from build123d import *

# Parameters (mm, degrees)
SKETCH001_W       = 214
SKETCH001_H       = 314
PAD_DEPTH         = 3
SKETCH_W          = 4
SKETCH_H          = 15
SKETCH_W_2        = 2
SKETCH_H_2        = 4
PAD001_DEPTH      = 0.3
SKETCH002_R       = 1.5
SKETCH002_R_2     = 0.75
POCKET_DEPTH      = 3.001
POCKET_DEPTH_BACK = -0.301


with BuildPart() as part:
    # Sketch001 → Pad (new body)
    with BuildSketch(Plane(origin=(110.543777, 322.172485, 403.912964), x_dir=(0, -1, 0), z_dir=(0, 0, 1))):
        with Locations((-107, 157)):
            Rectangle(SKETCH001_W, SKETCH001_H)
    extrude(amount=PAD_DEPTH)

    # Sketch → Pad001 (new body)
    with BuildSketch(Plane(origin=(110.543777, 322.172485, 406.912964), x_dir=(0, -1, 0), z_dir=(0, 0, 1))):
        with Locations((-208, 140)):
            Rectangle(SKETCH_W, SKETCH_H)
        with Locations((-208, 180)):
            Rectangle(SKETCH_W, SKETCH_H)
        with Locations((-208, 198)):
            Rectangle(SKETCH_W, SKETCH_H)
        with Locations((-210, 162.5)):
            Rectangle(SKETCH_W_2, SKETCH_H_2)
        with Locations((-207, 162.5)):
            Rectangle(SKETCH_W_2, SKETCH_H_2)
        with Locations((-208, 166.51)):
            Rectangle(SKETCH_W_2, SKETCH_H_2)
    extrude(amount=PAD001_DEPTH)

    # Sketch002 → Pocket (cut, two sides)
    with BuildSketch(Plane(origin=(110.543777, 322.172485, 406.912964), x_dir=(0, -1, 0), z_dir=(0, 0, 1))) as pocket_sk:
        with Locations((-208, 139.5)):
            Circle(SKETCH002_R)
        with Locations((-211, 157)):
            Circle(SKETCH002_R)
        with Locations((-210, 161.5)):
            Circle(SKETCH002_R_2)
        with Locations((-210, 163.5)):
            Circle(SKETCH002_R_2)
        with Locations((-207, 161.5)):
            Circle(SKETCH002_R_2)
        with Locations((-207, 163.5)):
            Circle(SKETCH002_R_2)
        with Locations((-208, 167.5)):
            Circle(SKETCH002_R_2)
        with Locations((-208, 165.5)):
            Circle(SKETCH002_R_2)
        with Locations((-208, 180.5)):
            Circle(SKETCH002_R)
        with Locations((-208, 197.5)):
            Circle(SKETCH002_R)
        with Locations((-211, 311)):
            Circle(SKETCH002_R)
        with Locations((-211, 3)):
            Circle(SKETCH002_R)
        with Locations((-3, 3)):
            Circle(SKETCH002_R)
        with Locations((-3, 311)):
            Circle(SKETCH002_R)
        with BuildLine():
            Line((-109.25, 159.250001), (-109.25, 153.25))
            Line((-109.25, 153.25), (-106.25, 153.25))
            Line((-106.25, 159.25), (-106.25, 153.25))
            ThreePointArc((-106.25, 159.25), (-107.75, 160.749999), (-109.25, 159.250001))
        make_face()
    extrude(amount=-POCKET_DEPTH, mode=Mode.SUBTRACT)
    extrude(pocket_sk.sketch, amount=-POCKET_DEPTH_BACK, mode=Mode.SUBTRACT)


solid = part.part
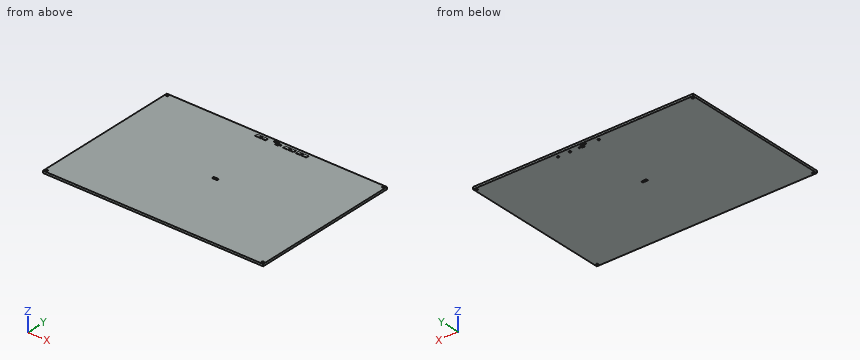
For this review, take the finished solid that the model builds, in its own axes (mm). Give positions to 0.01 mm unless a question says otherwise; leave off trailing zeros. Order: outer loops, then holes, each group sorted by start corner. A loop starts at its lowest first (then second) coordinate and runs counter-clockwise, first axis right, second up. Notation, with made-up numbers: M 34,46 L 84,46 A28 cw 84,70 Z; hole C 72,39 d3. An arc over 180 degrees is marked long. Answer in a Markdown table with one row per item. Add a question column.
(1) Consider section B-B on x = 199.5. State the section outline as (y, z) points, and give its area (3 significant figures).
(2) Wall thickness on probe 1 along Z at (x, y) = (160.5, 472): over which ranges is the line inside the solid? List them lowest first. Write a range as [from, to].
(3) Consider section A-A on y = 500.5. State the section outline as (x, z) points, and give its area (3 significant figures).
(4) For pin 1 (1.8 mm diameter, centred on x = 308.04, y = 530.17, fed in from -Z); pin 2 (1.5 mm diameter, centred on x = 372.5, y = 480, fed in from +Z), all flat-tipped, find the tip position at first contact; note any pin that passes through.
Evaluation:
| question | item | result |
|---|---|---|
| 1 | outline | M 322.17,403.91 L 536.17,403.91 L 536.17,406.91 L 322.17,406.91 Z |
| 1 | area | 642 mm^2 |
| 2 | probe 1 | z = [403.91, 406.91] |
| 3 | outline | M 110.54,403.91 L 424.54,403.91 L 424.54,406.91 L 110.54,406.91 Z |
| 3 | area | 942 mm^2 |
| 4 | pin 1 | passes through |
| 4 | pin 2 | stops at z = 406.91 |
